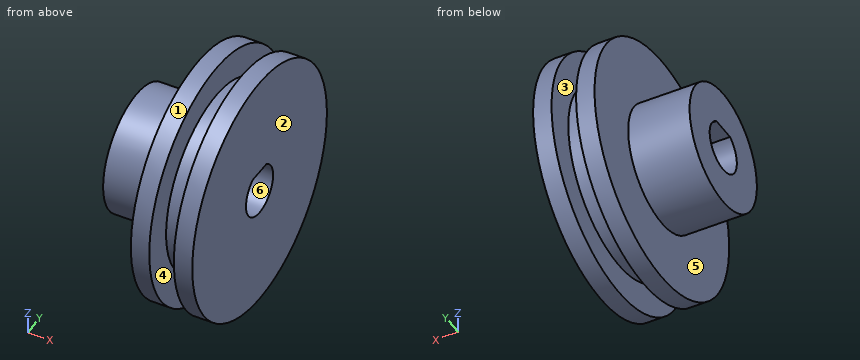
```python
from build123d import *

# Parameters (mm, degrees)
F0_R     = 25.4
F1_DEPTH = 6.35
F2_R     = 25.4
F2_R_2   = 19.05
F3_DEPTH = 2.54
F5_R     = 12.7
F6_DEPTH = 12.7
F7_DEPTH = 25.401


with BuildPart() as f1:
    # F0 (on Right) → F1 (new body, symmetric)
    with BuildSketch(Plane.YZ):
        Circle(F0_R)
    extrude(amount=F1_DEPTH, both=True)

    # F2 (on Right) → F3 (cut, symmetric)
    with BuildSketch(Plane.YZ):
        Circle(F2_R)
        Circle(F2_R_2, mode=Mode.SUBTRACT)
    extrude(amount=F3_DEPTH, both=True, mode=Mode.SUBTRACT)

    # F5 (on face) → F6 (join)
    with BuildSketch(Plane(origin=(-6.35, 0, 0), x_dir=(0, -1, 0), z_dir=(-1, 0, 0))):
        Circle(F5_R)
    extrude(amount=F6_DEPTH)

    # F4 (on face) → F7 (cut, through all)
    with BuildSketch(Plane.YZ.offset(6.35)):
        with BuildLine():
            Line((2.567312, 4.430939), (-2.567312, 4.430939))
            ThreePointArc((-2.567312, 4.430939), (0, -5.120968), (2.567312, 4.430939))
        make_face()
    extrude(amount=-F7_DEPTH, mode=Mode.SUBTRACT)


solid = f1.part
```
Here's how the part is built. I have some questions about the finished solid (model axes, mm). Face numbers are marked on the shaded views. A direction names the side the tool comes from. Give positions to 0.01 mm unless a question says otherwise; leave off trailing zeros. Write each loop counter-clockwise with the first axis right and the second up, starting at its lowest first coordinate (ties: lowest second). Pieces come first, ordered by that corner, then holes. Notation, with made-up numbers: M 14.5,23.5 L 46.5,23.5 A18 cw 46.5,38.5 Z; hole C 59.25,86.25 d5. An arc over 180 degrees is marked long. Put each result on its own line as item: value. Start each with the question number.
Item 1: If we section it at C-C, the plane x = -7: Write out the boundary of the cut face in (y, z).
Item 2: Thinking about a two-plate mould opening in X: for the marked faces 1, 2, 3 and 4, which applies, +X half, -X half, draft (parallel to the pull), parting line (faces both ways), or undercut?
Item 3: If we section it at B-B, the plane z = 0: Write out the boundary of the cut face in (x, y), then the cut area to 3 significant figures.
Item 4: If we section it at A-A, the plane y = 0: Write out the boundary of the cut face in (x, z), then the cut area to 3 significant figures.
Item 5: If we section it at D-D, the plane z = -20: Write out the boundary of the cut face in (x, y), then the cut area to 3 significant figures.
Item 6: Will these pins go through, and if not, where does the flat tip stop? pin 1 (10 mm diameter, centred on x = -8.5, z = 15, fed in from +Y); pin 2 (4 mm diameter, centred on x = -2, y = 9, fed in from -Z) (3 decimals); pin 3 (1 mm diameter, centred on x = -3.5, y = 6, fed in from +Z).
Item 7: On a 3-axis mill with a long thin cutter (end or side, diameter ignored), from which of +Z, -Z, +X, -X, +Y, -Y can I reach the whole of each face in a straight line? I mean the marked faces 5 and 6. Say none if no direction works.
Item 8: I need wall thicknesses on L1, parallel to X at y = 15, z = -18; L2, parallel to Z at x = -11.5, y = 0; L3, parallel to Z at x = -1.75, y = 0. Which ranges of each line are inside material? Lowest first, please. Write a range as from..to.
Values:
1. outline: C 0,0 d25.4; hole M -2.57,4.43 A5.12 ccw long 2.57,4.43 Z
2. face 1: draft
2. face 2: +X half
2. face 3: undercut
2. face 4: undercut
3. outline: M -19.05,-12.7 L -6.35,-12.7 L -6.35,-25.4 L -2.54,-25.4 L -2.54,-19.05 L 2.54,-19.05 L 2.54,-25.4 L 6.35,-25.4 L 6.35,-5.12 L -19.05,-5.12 Z; M -19.05,5.12 L 6.35,5.12 L 6.35,25.4 L 2.54,25.4 L 2.54,19.05 L -2.54,19.05 L -2.54,25.4 L -6.35,25.4 L -6.35,12.7 L -19.05,12.7 Z
3. area: 643 mm²
4. outline: M -19.05,-12.7 L -6.35,-12.7 L -6.35,-25.4 L -2.54,-25.4 L -2.54,-19.05 L 2.54,-19.05 L 2.54,-25.4 L 6.35,-25.4 L 6.35,-5.12 L -19.05,-5.12 Z; M -19.05,4.43 L 6.35,4.43 L 6.35,25.4 L 2.54,25.4 L 2.54,19.05 L -2.54,19.05 L -2.54,25.4 L -6.35,25.4 L -6.35,12.7 L -19.05,12.7 Z
4. area: 661 mm²
5. outline: M -6.35,-15.66 L -2.54,-15.66 L -2.54,15.66 L -6.35,15.66 Z; M 2.54,-15.66 L 6.35,-15.66 L 6.35,15.66 L 2.54,15.66 Z
5. area: 239 mm²
6. pin 1: y = 23.13
6. pin 2: z = -24.395
6. pin 3: z = 24.8
7. face 5: -X
7. face 6: +X, -X
8. L1: -6.35..-2.54, 2.54..6.35
8. L2: -12.7..-5.12, 4.43..12.7
8. L3: -19.05..-5.12, 4.43..19.05
